```python
from build123d import *

# Parameters (mm, degrees)
SKETCH1_W                = 30
SKETCH1_H                = 28.5
BOSS_EXTRUDE1_DEPTH      = 0.1
BOSS_EXTRUDE1_DEPTH_BACK = 3.15
SKETCH2_R                = 5
SKETCH2_R_2              = 1.3
CUT_EXTRUDE1_DEPTH       = 4.25
FILLET1_R                = 1.5


with BuildPart() as part:
    # Sketch1 → Boss-Extrude1 (new body, two sides)
    with BuildSketch(Plane(origin=(0, 0, 0), x_dir=(1, 0, 0), z_dir=(0, 1, 0))) as boss_extrude1_sk:
        Rectangle(SKETCH1_W, SKETCH1_H)
    extrude(amount=BOSS_EXTRUDE1_DEPTH)
    extrude(boss_extrude1_sk.sketch, amount=-BOSS_EXTRUDE1_DEPTH_BACK)

    # Sketch2 → Cut-Extrude1 (cut, through all)
    with BuildSketch(Plane(origin=(0, 0.1, 0), x_dir=(1, 0, 0), z_dir=(0, 1, 0))):
        Circle(SKETCH2_R)
        with Locations((0, 11)):
            Circle(SKETCH2_R_2)
        with Locations((7.778174593, 7.778174593)):
            Circle(SKETCH2_R_2)
        with Locations((11, 0)):
            Circle(SKETCH2_R_2)
        with Locations((7.778174593, -7.778174593)):
            Circle(SKETCH2_R_2)
        with Locations((0, -11)):
            Circle(SKETCH2_R_2)
        with Locations((-7.778174593, -7.778174593)):
            Circle(SKETCH2_R_2)
        with Locations((-11, 0)):
            Circle(SKETCH2_R_2)
        with Locations((-7.778174593, 7.778174593)):
            Circle(SKETCH2_R_2)
    extrude(amount=-CUT_EXTRUDE1_DEPTH, mode=Mode.SUBTRACT)

    # Fillet1
    fillet1_edges = [part.edges().sort_by_distance(p)[0] for p in [
        (-15, -1.525, -14.25),
        (15, -1.525, -14.25),
        (15, -1.525, 14.25),
        (-15, -1.525, 14.25),
    ]]
    fillet(fillet1_edges, radius=FILLET1_R)


solid = part.part
```
Could you check a few things on this model? Use its own coordinates, in mm. Round coordinates to 2 decimals unless told otherwise and drop trailing zeros. Write each loop counter-clockwise with the first axis right and the second up, starting at its lowest first coordinate (ties: lowest second). Pieces come first, ordered by that corner, then holes. Notation, with made-up numbers: M 57,62.25 L 71,62.25 A28 cw 71,99.25 Z; hole C 6.25,85 d9. An arc over 180 degrees is marked long. Answer in a Markdown table with one row per item. Add a question column.
Q1. If I drill on line 1 (Z direction, x = 0, y = -1.7); line 2 (Z direction, x = -0.5, y = -0.45); line 3 (Z direction, x = 7.25, y = -1.65), over which ranges is the centre line in solid material (lowest first)? Write a range as from..to.
Q2. If we mould it in two halves opening along X, with no side actions, what happens to faces 1 (the flat face through (15, -2, 0)), 2 (the cylindrical face through (-1.08, -1.5, 4.88)), 3 (the flat face through (0, -3.15, -7))? For each: +X half, -X half, draft (parallel to the pull), parting line (faces both ways), or undercut.
Q3. Imagine slicing it at C-C (z = -11). Please give me the cut outline in (x, y), then the cut area to 4 significant figures.
Q4. Imagine slicing it at D-D (y = -1.65). Give the number of separate pieces and of enclosed holes in the cut face, then the cut area to 3 significant figures.
Q5. Imagine slicing it at A-A (x = 0). Please give me the cut outline in (y, z).
Q6. Imagine slicing it at B-B (x = 11). Please give me the cut outline in (y, z).
Values:
| question | item | result |
|---|---|---|
| 1 | line 1 | -14.25..-12.3, -9.7..-5, 5..9.7, 12.3..14.25 |
| 1 | line 2 | -14.25..-12.2, -9.8..-4.97, 4.97..9.8, 12.2..14.25 |
| 1 | line 3 | -14.25..-8.97, -6.59..6.59, 8.97..14.25 |
| 2 | face 1 | +X half |
| 2 | face 2 | undercut |
| 2 | face 3 | draft |
| 3 | outline | M -15,-3.15 L -1.3,-3.15 L -1.3,0.1 L -15,0.1 Z; M 1.3,-3.15 L 15,-3.15 L 15,0.1 L 1.3,0.1 Z |
| 3 | area | 89.05 mm^2 |
| 4 | separate pieces | 1 |
| 4 | enclosed holes | 9 |
| 4 | area | 732 mm^2 |
| 5 | outline | M -3.15,-14.25 L 0.1,-14.25 L 0.1,-12.3 L -3.15,-12.3 Z; M -3.15,-9.7 L 0.1,-9.7 L 0.1,-5 L -3.15,-5 Z; M -3.15,5 L 0.1,5 L 0.1,9.7 L -3.15,9.7 Z; M -3.15,12.3 L 0.1,12.3 L 0.1,14.25 L -3.15,14.25 Z |
| 6 | outline | M -3.15,-14.25 L 0.1,-14.25 L 0.1,-1.3 L -3.15,-1.3 Z; M -3.15,1.3 L 0.1,1.3 L 0.1,14.25 L -3.15,14.25 Z |
